Verification items for the finished model (mm, model axes). A direction names the side the tool comes from. Round coordinates to 2 decimals unless told otherwise and drop trailing zeros. Write each loop counter-clockwise with the first axis right and the second up, starting at its lowest first coordinate (ties: lowest second). Pieces come first, ordered by that corner, then holes. Notation, with made-up numbers: (19, 7.25) -> (25, 7.25) arc R14 ccw to (25, 34.25) -> close; hole circle Ø9 at (64, 54.5). An arc over 180 degrees is marked (long way). Use CSV: the item, a comma, the result in double quotes.
```python
from build123d import *

# Parameters (mm, degrees)
EXTRUDE_1_DEPTH     = 3
SKETCH_2_R          = 1.35
CUT_EXTRUDE_1_DEPTH = 2.444444444
SKETCH_3_R          = 1.65
CUT_EXTRUDE_3_DEPTH = 96.756657889
CUT_EXTRUDE_4_DEPTH = 1


with BuildPart() as part:
    # 草图1 → 凸台-拉伸1 (new body)
    with BuildSketch(Plane.XY.offset(3)):
        with BuildLine():
            Line((-60.832535173, 7.514094179), (-91.218664305, 7.514094179))
            ThreePointArc((-91.218664305, 7.514094179), (-95.218664305, 3.514094179), (-91.218664305, -0.485905821))
            Line((-91.218664305, -0.485905821), (-60.531573746, -0.485905821))
            ThreePointArc((-60.531573746, -0.485905821), (-56.589491156, -2.306217172), (-52.451603626, -0.990377005))
            Line((-52.451603626, -0.990377005), (-50.420982545, -0.990377005))
            Line((-50.420982545, -0.990377005), (23.816560918, 0.467808699))
            Line((23.816560918, 0.467808699), (23.856567982, 0.468594524))
            ThreePointArc((23.856567982, 0.468594524), (27.777723532, 4.507000717), (23.778016459, 8.467622986))
            Line((23.778016459, 8.467622986), (-52.596358319, 8.467622986))
            ThreePointArc((-52.596358319, 8.467622986), (-56.905640848, 9.642312032), (-60.832535173, 7.514094179))
        make_face()
    extrude(amount=-EXTRUDE_1_DEPTH)

    # 草图2 → 切除-拉伸1 (cut)
    with BuildSketch(Plane.XY.offset(3)):
        with Locations(Location((23.77801746, 4.467622995, 0), (0, 0, 180))):
            Circle(SKETCH_2_R)
    extrude(amount=-CUT_EXTRUDE_1_DEPTH, mode=Mode.SUBTRACT)

    # 草图3 → 切除-拉伸3 (cut, through all)
    with BuildSketch(Plane(origin=(0, 0, 0), x_dir=(-1, 0, 0), z_dir=(0, 0, -1))):
        with Locations(Location((-23.778017455, 4.467823177, 0), (0, 0, 180))):
            Circle(SKETCH_3_R)
        with Locations((56.215610459, 3.6821226)):
            Circle(SKETCH_3_R)
        with Locations((91.218664305, 3.514094179)):
            Circle(SKETCH_3_R)
    extrude(amount=-CUT_EXTRUDE_3_DEPTH, mode=Mode.SUBTRACT)

    # 草图4 → 切除-拉伸4 (cut)
    with BuildSketch(Plane(origin=(0, 0, 0), x_dir=(-1, 0, 0), z_dir=(0, 0, -1))):
        with BuildLine():
            Line((80.04205053, 5.564500073), (80.04205053, 5.205525714))
            Line((80.04205053, 5.205525714), (78.851545722, 5.205525714))
            Line((78.851545722, 5.205525714), (78.662943959, 4.284952797))
            add(Edge.make_bspline(
                [(78.662943959, 4.284952797), (78.699999834, 4.295183069), (78.77178973, 4.315002603), (78.877749591, 4.337008373), (78.978341794, 4.350273817), (79.043617164, 4.352085128), (79.075203575, 4.352961612)],
                knots=[0, 0, 0, 0, 1.100273476, 2.13160584, 3.095893838, 4, 4, 4, 4], degree=3))
            add(Edge.make_bspline(
                [(79.075203575, 4.352961612), (79.114287314, 4.352115676), (79.191135712, 4.350452355), (79.303574659, 4.334480505), (79.410907552, 4.309340591), (79.512909922, 4.274220069), (79.609770473, 4.229310336), (79.700598034, 4.173210396), (79.786755947, 4.107677064), (79.866698541, 4.032332052), (79.939222849, 3.949410436), (80.002988839, 3.860252565), (80.057151429, 3.765724903), (80.100712184, 3.664924294), (80.135496519, 3.55896514), (80.158648513, 3.446732558), (80.174065222, 3.329284438), (80.175787609, 3.248979868), (80.176665915, 3.208029721)],
                knots=[0, 0, 0, 0, 1.052922333, 2.070308379, 3.05430497, 4.020497103, 4.973039431, 5.925935799, 6.892292201, 7.88610001, 8.88166317, 9.857072816, 10.836096531, 11.812156883, 12.81219415, 13.836441305, 14.89672472, 16, 16, 16, 16], degree=3))
            add(Edge.make_bspline(
                [(80.176665915, 3.208029721), (80.176000839, 3.1795075), (80.174679677, 3.122848513), (80.167961089, 3.038704312), (80.155025373, 2.956341479), (80.137657649, 2.875749087), (80.115115231, 2.797079715), (80.087826177, 2.720108187), (80.054430149, 2.64531358), (80.017798774, 2.571988185), (79.976552296, 2.501789678), (79.930773789, 2.436140691), (79.882408298, 2.37405641), (79.830366912, 2.316202677), (79.774165917, 2.262959659), (79.71448595, 2.214011377), (79.651803231, 2.168530047), (79.585147989, 2.128361852), (79.516005506, 2.091398896), (79.443377289, 2.061075359), (79.368916588, 2.03396483), (79.291551713, 2.012355303), (79.2114579, 1.995422748), (79.128503125, 1.983922148), (79.043122455, 1.97554571), (78.985247442, 1.975021353), (78.95601287, 1.974756483)],
                knots=[0, 0, 0, 0, 1.056347294, 2.098418968, 3.122841568, 4.141288669, 5.149314143, 6.15115421, 7.162517403, 8.180376062, 9.185164535, 10.17417709, 11.141909838, 12.097768115, 13.052685741, 14.0056014, 14.954263652, 15.917497458, 16.885230207, 17.854509472, 18.828990115, 19.81800267, 20.826176721, 21.857883937, 22.917946725, 24, 24, 24, 24], degree=3))
            add(Edge.make_bspline(
                [(78.95601287, 1.974756483), (78.921138689, 1.975447321), (78.852527858, 1.976806463), (78.752007291, 1.991024949), (78.655292685, 2.011388865), (78.563162584, 2.042025135), (78.474791321, 2.08041243), (78.391368603, 2.128928601), (78.310762827, 2.183907705), (78.23625079, 2.248788058), (78.167094677, 2.31970374), (78.105188168, 2.396661381), (78.050054591, 2.478390823), (78.002576844, 2.565288977), (77.962078823, 2.657127508), (77.930263834, 2.754250509), (77.904585479, 2.856150513), (77.893722059, 2.926304023), (77.888204376, 2.961935971)],
                knots=[0, 0, 0, 0, 1.0467383, 2.05933395, 3.04377827, 4.011590433, 4.970194871, 5.932262533, 6.905835911, 7.896367577, 8.894135286, 9.877477877, 10.858688626, 11.851381753, 12.8477658, 13.868841284, 14.917554742, 16, 16, 16, 16], degree=3))
            Line((77.888204376, 2.961935971), (78.20230694, 2.961935971))
            add(Edge.make_bspline(
                [(78.20230694, 2.961935971), (78.210035498, 2.928559518), (78.224890214, 2.864408123), (78.257495963, 2.774276782), (78.297361838, 2.693957558), (78.344766187, 2.622387975), (78.401316217, 2.559978978), (78.465845646, 2.504361916), (78.538193369, 2.454186786), (78.618586599, 2.412364019), (78.703399678, 2.376695266), (78.792166888, 2.352943571), (78.882471235, 2.336242678), (78.943549605, 2.334570917), (78.974242036, 2.333730842)],
                knots=[0, 0, 0, 0, 1.136247022, 2.183929868, 3.172523383, 4.106158343, 5.02341133, 5.958108904, 6.928429099, 7.938127109, 8.96079061, 9.975095812, 10.982467395, 12, 12, 12, 12], degree=3))
            add(Edge.make_bspline(
                [(78.974242036, 2.333730842), (79.004200481, 2.33455162), (79.063188903, 2.336167739), (79.15000029, 2.348606751), (79.233813164, 2.367764322), (79.313800521, 2.396434177), (79.39136206, 2.431278895), (79.464535831, 2.475993971), (79.535438708, 2.52745399), (79.601866841, 2.58641062), (79.662706291, 2.651380314), (79.716462412, 2.720857708), (79.761239325, 2.794974554), (79.798973434, 2.872447707), (79.827626733, 2.954126264), (79.848067714, 3.03962744), (79.860070773, 3.12916242), (79.861721953, 3.19023173), (79.86256335, 3.221351035)],
                knots=[0, 0, 0, 0, 1.027316725, 2.022795036, 3.002884548, 3.971462791, 4.93288096, 5.914575861, 6.907176829, 7.935150275, 8.956128384, 9.956726525, 10.942570165, 11.921478529, 12.907843606, 13.90538589, 14.932640048, 16, 16, 16, 16], degree=3))
            add(Edge.make_bspline(
                [(79.86256335, 3.221351035), (79.861904871, 3.249426786), (79.860615991, 3.304381075), (79.850085421, 3.384780282), (79.831768448, 3.460853324), (79.806344569, 3.532967558), (79.774065061, 3.601191), (79.734618748, 3.665594061), (79.687265351, 3.725327894), (79.633173462, 3.780420447), (79.573915421, 3.831265322), (79.508471678, 3.874609409), (79.438211752, 3.911073326), (79.363982152, 3.942541325), (79.284017254, 3.96514207), (79.199900621, 3.982109956), (79.110723913, 3.991925318), (79.049753225, 3.993287207), (79.018412709, 3.993987253)],
                knots=[0, 0, 0, 0, 1.045622112, 2.046656509, 3.013763289, 3.955457236, 4.890082067, 5.820317437, 6.762574623, 7.722996705, 8.69280354, 9.665887285, 10.63943826, 11.638615906, 12.663482002, 13.728887084, 14.832589034, 16, 16, 16, 16], degree=3))
            add(Edge.make_bspline(
                [(79.018412709, 3.993987253), (78.991283781, 3.993406661), (78.935269425, 3.992207888), (78.849346599, 3.983381391), (78.759054876, 3.969142097), (78.66474038, 3.949555849), (78.566119872, 3.923924772), (78.463401471, 3.893210272), (78.356369205, 3.856488273), (78.28425148, 3.828756059), (78.247178735, 3.814500073)],
                knots=[0, 0, 0, 0, 0.817624296, 1.688186739, 2.600797293, 3.572016777, 4.590301741, 5.671205678, 6.80286297, 8, 8, 8, 8], degree=3))
            Line((78.247178735, 3.814500073), (78.606153094, 5.564500073))
            Line((78.606153094, 5.564500073), (80.04205053, 5.564500073))
        make_face()
    extrude(amount=-CUT_EXTRUDE_4_DEPTH, mode=Mode.SUBTRACT)


solid = part.part
```
Q1. Section check C-C (x = 2.5). Record the cut outline in (y, z).
Filled in:
outline,"(0.05, 0) -> (8.47, 0) -> (8.47, 3) -> (0.05, 3) -> close"
Q2. Section check B-B (x = -85). Record the cut outline in (y, z).
Filled in:
outline,"(-0.49, 0) -> (7.51, 0) -> (7.51, 3) -> (-0.49, 3) -> close"
Q3. Mould release check, pull along X, two halves, no side actions. Record for faces 6 (the flat face through (-14, 8.468, 2)), 7 (the cylindrical face through (-54.567, 3.755, 1.479)), 8 (the cylindrical face through (-56.84, 9.65, 1.52)): released by +X, released by -X, zero draft, split by the parting line, or undercut.
Filled in:
face 6,"zero draft"
face 7,"undercut"
face 8,"split by the parting line"
Q4. Material ranges on L1, parallel to X at y = 2.25, z = 0.85; L2, parallel to X at y = 2, z = 1.45; L3, parallel to Y at x = -63, z = 0.65, recorded low to high.
Filled in:
L1,"-95.01 to -92.28, -90.16 to -79.76, -78.24 to -57.04, -55.4 to 27.11"
L2,"-94.92 to -91.87, -90.56 to 26.93"
L3,"-0.49 to 7.51"
Q5. Section check A-A (z = 2.5). Record the cut outline in (x, y).
Filled in:
outline,"(-91.22, -0.49) -> (-60.53, -0.49) arc R6 ccw to (-52.45, -0.99) -> (-50.42, -0.99) -> (23.86, 0.47) arc R4 ccw to (23.78, 8.47) -> (-52.6, 8.47) arc R6 ccw to (-60.83, 7.51) -> (-91.22, 7.51) arc R4 ccw to start; hole circle Ø3.3 at (-91.22, 3.51); hole circle Ø3.3 at (-56.22, 3.68); hole circle Ø3.3 at (23.78, 4.47)"
Q6. Go/stop test with flat-tipped pins: P1, Ø2.5, axis at x = -78.5, y = 3.5, coming from the -Z side; P2, Ø1.5, axis at x = -68.5, z = 1.5, coming from the +Y side. Record where each tip stops, or that it passes through.
Filled in:
P1,"z = 0"
P2,"y = 7.51"
Q7. Access from +Z, -Z, +X, -X, +Y, -Y to the whole of each face (thin tool, end or side, straight path). Record for faces 1 (the flat face through (-35, 4, 0)), 2 (the flat face through (-51, -0.99, 2)), 3 (the flat face through (-35, 4, 3)), 4 (the flat face through (-76, -0.486, 2)), 5 (the flat face through (-76, 7.514, 2)).
Filled in:
face 1,"-Z, +X, -X, +Y, -Y"
face 2,"+Z, -Z, +X, -Y"
face 3,"+Z, +X, -X, +Y, -Y"
face 4,"+Z, -Z, -X, -Y"
face 5,"+Z, -Z, -X, +Y"
